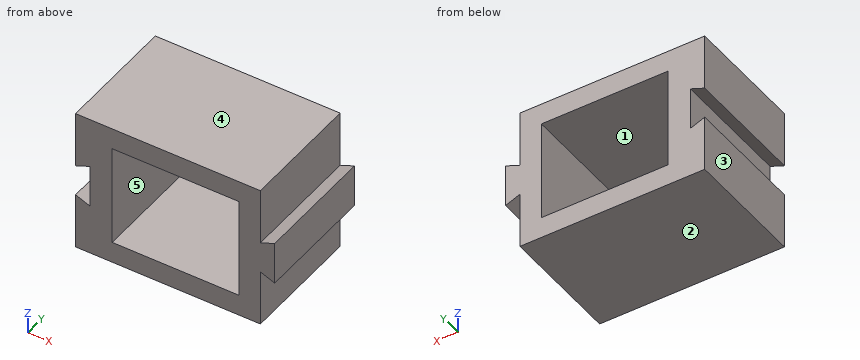
from build123d import *

# Parameters (mm, degrees)
BOSS_EXTRUDE1_DEPTH = 42.5
SKETCH2_W           = 44.214702114
SKETCH2_H           = 35.5
CUT_EXTRUDE1_DEPTH  = 42.5


with BuildPart() as part:
    # Sketch1 → Boss-Extrude1 (new body)
    with BuildSketch(Plane(origin=(0, 0, 0), x_dir=(1, 0, 0), z_dir=(0, 1, 0))):
        Polygon((-32.25, 25.25), (-32.25, 5.5), (-27.25, 7.5), (-27.25, -7.5), (-32.25, -5.5), (-32.25, -25.25), (32.25, -25.25), (32.25, -5.5), (32.25, 5.5), (32.25, 25.25), align=None)
        Polygon((37.25, 7.5), (32.25, 5.5), (32.25, -5.5), (37.25, -7.5), align=None)
    extrude(amount=BOSS_EXTRUDE1_DEPTH)

    # Sketch2 → Cut-Extrude1 (cut)
    with BuildSketch(Plane(origin=(0, 42.5, 0), x_dir=(1, 0, 0), z_dir=(0, 1, 0))):
        with Locations((2.642648943, 0)):
            Rectangle(SKETCH2_W, SKETCH2_H)
    extrude(amount=-CUT_EXTRUDE1_DEPTH, mode=Mode.SUBTRACT)


solid = part.part
Could you check a few things on this model? Use its own coordinates, in mm. Face numbers are marked on the shaded views. A direction names the side the tool comes from. Give positions to 0.01 mm unless a question says otherwise; leave off trailing zeros. Loops run counter-clockwise (first coordinate to the right, second up) from the corner with the lowest first, then second, coordinate; pieces in that order, holes last. Notation, with made-up numbers: M 9.25,46 L 59.25,46 A29 ccw 59.25,81 Z; hole C 68.25,5.25 d7. An arc over 180 degrees is marked long. Answer as a JSON object with one key per item and string values.
Q1. Suppose I cut it at D-D, the plane z = -20.5. List the corners of the cut face in (x, y) for me.
Values found:
{"outline": "M -32.25,0 L 32.25,0 L 32.25,42.5 L -32.25,42.5 Z"}
Q2. For P1, Ø1, axis at y = 32, z = 9.5, coming from the +X side; P2, Ø4.5, axis at y = 16, z = -1.5, coming from the -X side; P3, Ø8, axis at x = 17, z = -9.5, coming from the -Y side, each with a flat end and sliding along its axis, tell me the tip position at first contact or that it passes through.
Values found:
{"P1": "stops at x = 32.25", "P2": "stops at x = -27.25", "P3": "passes through"}
Q3. For the marked faces 1 and 2, which set-ups out of +Z, -Z, +X, -X, +Y, -Y let a thin tool reach every point of the face, with its end or its side?
Values found:
{"face 1": "+Y, -Y", "face 2": "-Z, +X, -X, +Y, -Y"}
Q4. If we mould it in two halves opening along Z, with no side actions, what happens to the marked faces 3, 4 and 5? For each: pulls with the +Z half, pulls with the -Z half, needs draft (parallel to the pull), parting line crosses it, or undercut.
Values found:
{"face 3": "needs draft", "face 4": "pulls with the +Z half", "face 5": "undercut"}
Q5. Suppose I cut it at B-B, the plane z = -11.5. List the corners of the cut face in (x, y) for me, plus the area to 3 significant figures.
Values found:
{"outline": "M -32.25,0 L -19.46,0 L -19.46,42.5 L -32.25,42.5 Z; M 24.75,0 L 32.25,0 L 32.25,42.5 L 24.75,42.5 Z", "area": "862 mm²"}
Q6. Suppose I cut it at C-C, the plane x = 8.5. List the corners of the cut face in (y, z) for me.
Values found:
{"outline": "M 0,-25.25 L 42.5,-25.25 L 42.5,-17.75 L 0,-17.75 Z; M 0,17.75 L 42.5,17.75 L 42.5,25.25 L 0,25.25 Z"}
Q7. Suppose I cut it at A-A, the plane y = 16.5. List the corners of the cut face in (x, z) for me.
Values found:
{"outline": "M -32.25,-25.25 L 32.25,-25.25 L 32.25,-5.5 L 37.25,-7.5 L 37.25,7.5 L 32.25,5.5 L 32.25,25.25 L -32.25,25.25 L -32.25,5.5 L -27.25,7.5 L -27.25,-7.5 L -32.25,-5.5 Z; hole M -19.46,-17.75 L 24.75,-17.75 L 24.75,17.75 L -19.46,17.75 Z"}
Q8. If I drill on probe 1 along Z at (x, y) = (-10, 34); probe 2 along X at (y, z) = (2, 17); probe 3 along X at (y, z) = (21.5, 3.5), over which ranges is the centre line in solid material (lowest first)? Write a range as [from, to].
Values found:
{"probe 1": "z = [-25.25, -17.75], [17.75, 25.25]", "probe 2": "x = [-32.25, -19.46], [24.75, 32.25]", "probe 3": "x = [-27.25, -19.46], [24.75, 37.25]"}
